Here's how the part is built. I have some questions about the finished solid (model axes, mm). Face numbers are marked on the shaded views. A direction names the side the tool comes from. Round coordinates to 2 decimals unless told otherwise and drop trailing zeros. Order: outer loops, then holes, each group sorted by start corner. A loop starts at its lowest first (then second) coordinate and runs counter-clockwise, first axis right, second up. Notation, with made-up numbers: (-1.75, 85) -> (35.25, 85) arc R28 ccw to (35.25, 106) -> close; hole circle Ø1 at (54, -10.5). An arc over 180 degrees is marked (long way). Use a Markdown table: item, result. Add a question column.
(1) Thinking about a two-plate mould opening in Y: for the marked faces 1, 2 and 3, which applies, pulls with the +Y half, pulls with the -Y half, needs draft (parallel to the pull), parting line crosses it, or undercut?
(2) If I drill on probe 1 along Y at (x, z) = (34, 27.5); probe 2 along Y at (x, z) = (-58, 16); probe 3 along Y at (x, z) = (53, 32), over which ranges is the centre line in solid material (lowest first)?
(3) I want a section at A-A, the plane z = 17. Please give me the cut outline in (x, y), then the cut area to 3 significant figures.
(4) I want a section at C-C, the plane x = 25.5. Please give me the cut outline in (y, z).
(5) I'm going to push flat-ended pins straight in: P1, Ø5, axis at y = 66, z = 16.5, coming from the +X side; P2, Ø5, axis at x = 65, z = 16, coming from the +Y side; P3, Ø10.5, axis at x = 62.5, y = -24.5, coming from the -Z side; P4, Ø3, axis at y = -69, z = 11.5, coming from the +X side. Where does each tip first touch, or does it pass through?
(6) I want a section at D-D, the plane z = 27. Please give me the cut outline in (x, y).
(7) I want a section at B-B, the plane y = 37.5. Please give me the cut outline in (x, z), then the cut area to 3 significant figures.
(8) On a 3-axis mill with a long thin cutter (end or side, diameter ignored), from which of +Z, -Z, +X, -X, +Y, -Y can I reach the whole of each face in a straight line? I mean the marked faces 4 and 5. Say none if no direction works.
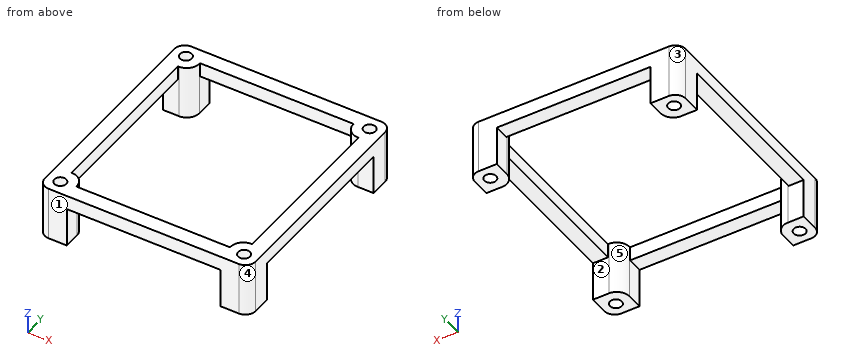
from build123d import *

# Parameters (mm, degrees)
F0_W     = 114
F0_H     = 124
F1_DEPTH = 34
F2_W     = 97
F2_H     = 42.713016
F2_W_2   = 43.496885
F2_H_2   = 107
F2_W_3   = 85.450368
F2_H_3   = 43.636596
F3_DEPTH = 25
F4_R     = 3.75
F5_DEPTH = 34
F6_DEPTH = 34


with BuildPart() as f1:
    # F0 (on Top) → F1 (new body)
    with BuildSketch(Plane.XY):
        with BuildLine():
            ThreePointArc((-65.365605, -65.46179), (-63.461799, -70.057984), (-58.865605, -71.96179))
            Line((-58.865605, -71.96179), (61.134395, -71.96179))
            ThreePointArc((61.134395, -71.96179), (65.730589, -70.057984), (67.634395, -65.46179))
            Line((67.634395, -65.46179), (67.634395, 64.53821))
            ThreePointArc((67.634395, 64.53821), (65.730589, 69.134404), (61.134395, 71.03821))
            Line((61.134395, 71.03821), (-58.865605, 71.03821))
            ThreePointArc((-58.865605, 71.03821), (-63.461799, 69.134404), (-65.365605, 64.53821))
            Line((-65.365605, 64.53821), (-65.365605, -65.46179))
        make_face()
        with Locations((1.134395, -0.46179)):
            Rectangle(F0_W, F0_H, mode=Mode.SUBTRACT)
    extrude(amount=F1_DEPTH)

    # F2 (on face) → F3 (cut)
    with BuildSketch(Plane(origin=(0, 0, 0), x_dir=(1, 0, 0), z_dir=(0, 0, -1))):
        with Locations((1.134395, 75.318298)):
            Rectangle(F2_W, F2_H)
        with Locations((-69.114047, 0.46179)):
            Rectangle(F2_W_2, F2_H_2)
        with Locations((92.359579, 0.46179)):
            Rectangle(F2_W_3, F2_H_2)
        with Locations((1.134395, -74.856508)):
            Rectangle(F2_W, F2_H_3)
    extrude(amount=-F3_DEPTH, mode=Mode.SUBTRACT)

    # F4 (on Top) → F5 (join)
    with BuildSketch(Plane.XY):
        with BuildLine():
            ThreePointArc((-47.365605, -61.96179), (-49.708751, -56.304936), (-55.365605, -53.96179))
            Line((-55.365605, -53.96179), (-65.365605, -53.96179))
            Line((-65.365605, -53.96179), (-65.365605, -65.46179))
            ThreePointArc((-65.365605, -65.46179), (-63.461799, -70.057984), (-58.865605, -71.96179))
            Line((-58.865605, -71.96179), (-47.365605, -71.96179))
            Line((-47.365605, -71.96179), (-47.365605, -61.96179))
        make_face()
        with Locations((-56.865605, -63.46179)):
            Circle(F4_R, mode=Mode.SUBTRACT)
        with BuildLine():
            ThreePointArc((57.634395, -53.96179), (51.977541, -56.304936), (49.634395, -61.96179))
            Line((49.634395, -61.96179), (49.634395, -71.96179))
            Line((49.634395, -71.96179), (61.134395, -71.96179))
            ThreePointArc((61.134395, -71.96179), (65.730589, -70.057984), (67.634395, -65.46179))
            Line((67.634395, -65.46179), (67.634395, -53.96179))
            Line((67.634395, -53.96179), (57.634395, -53.96179))
        make_face()
        with Locations((59.134395, -63.46179)):
            Circle(F4_R, mode=Mode.SUBTRACT)
        with BuildLine():
            Line((57.634395, 53.03821), (67.634395, 53.03821))
            Line((67.634395, 53.03821), (67.634395, 64.53821))
            ThreePointArc((67.634395, 64.53821), (65.730589, 69.134404), (61.134395, 71.03821))
            Line((61.134395, 71.03821), (49.634395, 71.03821))
            Line((49.634395, 71.03821), (49.634395, 61.03821))
            ThreePointArc((49.634395, 61.03821), (51.977541, 55.381355), (57.634395, 53.03821))
        make_face()
        with Locations((59.134395, 62.53821)):
            Circle(F4_R, mode=Mode.SUBTRACT)
        with BuildLine():
            Line((-65.365605, 53.03821), (-55.365605, 53.03821))
            ThreePointArc((-55.365605, 53.03821), (-49.708751, 55.381355), (-47.365605, 61.03821))
            Line((-47.365605, 61.03821), (-47.365605, 71.03821))
            Line((-47.365605, 71.03821), (-58.865605, 71.03821))
            ThreePointArc((-58.865605, 71.03821), (-63.461799, 69.134404), (-65.365605, 64.53821))
            Line((-65.365605, 64.53821), (-65.365605, 53.03821))
        make_face()
        with Locations((-56.865605, 62.53821)):
            Circle(F4_R, mode=Mode.SUBTRACT)
    extrude(amount=F5_DEPTH)

    # F4 (on Top) → F6 (cut)
    with BuildSketch(Plane.XY):
        with Locations((-56.865605, -63.46179)):
            Circle(F4_R)
        with Locations((59.134395, -63.46179)):
            Circle(F4_R)
        with Locations((59.134395, 62.53821)):
            Circle(F4_R)
        with Locations((-56.865605, 62.53821)):
            Circle(F4_R)
    extrude(amount=F6_DEPTH, mode=Mode.SUBTRACT)


solid = f1.part
Taken from the geometry:
| question | item | result |
|---|---|---|
| 1 | face 1 | pulls with the -Y half |
| 1 | face 2 | undercut |
| 1 | face 3 | pulls with the +Y half |
| 2 | probe 1 | y = -71.96 to -62.46, 61.54 to 71.04 |
| 2 | probe 2 | y = -71.96 to -67.04, -59.89 to -53.96, 53.04 to 58.96, 66.11 to 71.04 |
| 2 | probe 3 | y = -71.96 to -55.44, 54.52 to 71.04 |
| 3 | outline | (-65.37, -65.46) arc R6.5 ccw to (-58.87, -71.96) -> (-47.37, -71.96) -> (-47.37, -61.96) arc R8 ccw to (-55.37, -53.96) -> (-65.37, -53.96) -> close; (-65.37, 53.04) -> (-55.37, 53.04) arc R8 ccw to (-47.37, 61.04) -> (-47.37, 71.04) -> (-58.87, 71.04) arc R6.5 ccw to (-65.37, 64.54) -> close; (49.63, -71.96) -> (61.13, -71.96) arc R6.5 ccw to (67.63, -65.46) -> (67.63, -53.96) -> (57.63, -53.96) arc R8 ccw to (49.63, -61.96) -> close; (49.63, 61.04) arc R8 ccw to (57.63, 53.04) -> (67.63, 53.04) -> (67.63, 64.54) arc R6.5 ccw to (61.13, 71.04) -> (49.63, 71.04) -> close; hole circle Ø7.5 at (-56.87, -63.46); hole circle Ø7.5 at (-56.87, 62.54); hole circle Ø7.5 at (59.13, -63.46); hole circle Ø7.5 at (59.13, 62.54) |
| 3 | area | 1,030 mm2 |
| 4 | outline | (-71.96, 25) -> (-62.46, 25) -> (-62.46, 34) -> (-71.96, 34) -> close; (61.54, 25) -> (71.04, 25) -> (71.04, 34) -> (61.54, 34) -> close |
| 5 | P1 | stops at x = 67.63 |
| 5 | P2 | stops at y = 70.89 |
| 5 | P3 | stops at z = 25 |
| 5 | P4 | stops at x = 67.31 |
| 6 | outline | (-65.37, -65.46) arc R6.5 ccw to (-58.87, -71.96) -> (61.13, -71.96) arc R6.5 ccw to (67.63, -65.46) -> (67.63, 64.54) arc R6.5 ccw to (61.13, 71.04) -> (-58.87, 71.04) arc R6.5 ccw to (-65.37, 64.54) -> close; hole circle Ø7.5 at (-56.87, -63.46); hole circle Ø7.5 at (-56.87, 62.54); hole (-55.87, -53.96) -> (-55.37, -53.96) arc R8 cw to (-47.37, -61.96) -> (-47.37, -62.46) -> (49.63, -62.46) -> (49.63, -61.96) arc R8 cw to (57.63, -53.96) -> (58.13, -53.96) -> (58.13, 53.04) -> (57.63, 53.04) arc R8 cw to (49.63, 61.04) -> (49.63, 61.54) -> (-47.37, 61.54) -> (-47.37, 61.04) arc R8 cw to (-55.37, 53.04) -> (-55.87, 53.04) -> close; hole circle Ø7.5 at (59.13, -63.46); hole circle Ø7.5 at (59.13, 62.54) |
| 7 | outline | (-65.37, 25) -> (-55.87, 25) -> (-55.87, 34) -> (-65.37, 34) -> close; (58.13, 25) -> (67.63, 25) -> (67.63, 34) -> (58.13, 34) -> close |
| 7 | area | 171 mm2 |
| 8 | face 4 | +Z, -Z, +X, -Y |
| 8 | face 5 | +Z, -Z |
